Check sheet for the modelled part. Datum: model origin and axes. Units: mm. A direction names the side the tool comes from. Give positions to 0.01 mm unless a question says otherwise; leave off trailing zeros. Order: outer loops, then holes, each group sorted by start corner. A loop starts at its lowest first (then second) coordinate and runs counter-clockwise, first axis right, second up.
```python
from build123d import *

# Parameters (mm, degrees)
SKETCH_1_R      = 24.5
EXTRUDE_1_DEPTH = 4
SKETCH_2_W      = 4
SKETCH_2_H      = 45
EXTRUDE_2_DEPTH = 2
SKETCH_3_R      = 1.75
EXTRUDE_3_DEPTH = 3
FILLET_2_R      = 1.7


with BuildPart() as part:
    # 草图1 → 凸台-拉伸1 (new body)
    with BuildSketch(Plane.XY):
        Circle(SKETCH_1_R)
    extrude(amount=EXTRUDE_1_DEPTH)

    # 草图2 → 凸台-拉伸2 (add)
    with BuildSketch(Plane.XY.offset(4)):
        Rectangle(SKETCH_2_W, SKETCH_2_H)
    extrude_2 = extrude(amount=EXTRUDE_2_DEPTH)

    # 镜向1: 凸台-拉伸2 across plane
    add(extrude_2.mirror(Plane.XY.offset(2)))

    # 草图3 → 凸台-拉伸3 (add)
    with BuildSketch(Plane(origin=(0, -24, 0), x_dir=(-1, 0, 0), z_dir=(0, -1, 0))):
        with Locations(Location((0, -2, 0), (0, 0, 270))):
            Circle(SKETCH_3_R)
    extrude(amount=EXTRUDE_3_DEPTH)

    # 圆角2
    fillet_2_edges = [part.edges().sort_by_distance(p)[0] for p in [
        (0, -27, 0.25),
    ]]
    fillet(fillet_2_edges, radius=FILLET_2_R)


solid = part.part
```
(1) Material ranges on L1, parallel to Z at x = 11, y = -10; L2, parallel to X at y = 3, z = -0.75; L3, parallel to Y at x = 13, z = 0.25, recorded low to high.
Response values:
L1: z = 0 to 4
L2: x = -2 to 2
L3: y = -20.77 to 20.77
(2) Cross-section at A-A on y = 0. Enter the section's corners in (x, z).
Response values:
outline: (-24.5, 0) - (-2, 0) - (-2, -2) - (2, -2) - (2, 0) - (24.5, 0) - (24.5, 4) - (2, 4) - (2, 6) - (-2, 6) - (-2, 4) - (-24.5, 4) - close
(3) Cross-section at C-C on x = 8. Enter the section's corners in (y, z).
Response values:
outline: (-23.16, 0) - (23.16, 0) - (23.16, 4) - (-23.16, 4) - close
(4) Set-up check for faces 1 (the face through (0, 22.5, -1)), 2 (the face through (0, -22.5, -1)), 3 (the face through (2, 0, 5)), 4 (the face through (2, 0, -1)), 5 (the face through (0, -22.5, 5)): record each of +Z, -Z, +X, -X, +Y, -Y from which the full face is reachable in a straight line by a thin tool's end or side.
Response values:
face 1: -Z, +X, -X, +Y
face 2: -Z, +X, -X, -Y
face 3: +Z, +X, +Y, -Y
face 4: -Z, +X, +Y, -Y
face 5: +Z, +X, -X, -Y
(5) Cross-section at B-B on z = -1.25. Enter the section's corners in (x, y).
Response values:
outline: (-2, -22.5) - (2, -22.5) - (2, 22.5) - (-2, 22.5) - close
(6) Cross-section at D-D on y = -21. Enter the section's corners in (x, z).
Response values:
outline: (-12.62, 0) - (-2, 0) - (-2, -2) - (2, -2) - (2, 0) - (12.62, 0) - (12.62, 4) - (2, 4) - (2, 6) - (-2, 6) - (-2, 4) - (-12.62, 4) - close
(7) Gauge pin test, flat ends, axial feed: pin 1 Ø1 at (x, z) = (1, 5.5) entering from +Y; pin 2 Ø8 at (x, y) = (16.5, 13.5) entering from +Z; pin 3 Ø0.6 at (x, z) = (0, -1) entering from -Y. Record the tip position at first contact, or that the pin passes through.
Response values:
pin 1: stops at y = 22.5
pin 2: stops at z = 4
pin 3: stops at y = -22.5
